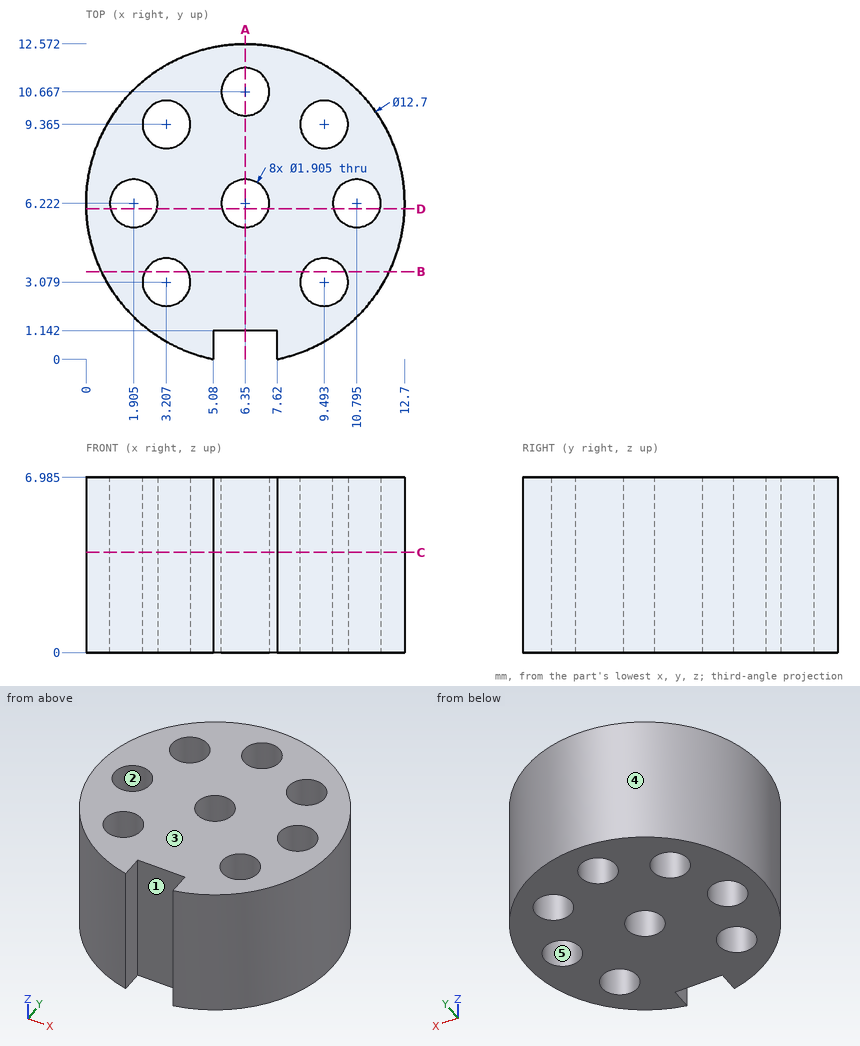
Can you work these out from the drawing? Everything is in mm from the part's minimum corner. A direction names the side the tool comes from. Give positions to 0.01 mm unless a question says otherwise; leave off trailing zeros. Order: outer loops, then holes, each group sorted by start corner. A loop starts at its lowest first (then second) coordinate and runs counter-clockwise, first axis right, second up. Notation, with made-up numbers: M 47.25,32.5 L 80.25,32.5 A19 ccw 80.25,59.5 Z; hole C 28,10 d4. An arc over 180 degrees is marked long. One line per question, with ' | ' between items.
1. For the marked faces 1 and 2, which set-ups out of +Z, -Z, +X, -X, +Y, -Y let a thin tool reach every point of the face, with its end or its side?
Results:
face 1: +Z, -Z, -Y | face 2: +Z, -Z
2. I want a section at C-C (z = 4). Give the number of separate pieces and of enclosed holes in the cut face, and give its area (3 significant figures).
Results:
separate pieces: 1 | enclosed holes: 8 | area: 101 mm²
3. We'd pull the mould along X, two halves only. Please class the marked faces 3, 4 and 5: +X half, -X half, draft (parallel to the pull), parting line (faces both ways), or undercut.
Results:
face 3: draft | face 4: parting line | face 5: undercut
4. If I drill on line 1 (Y direction, x = 6.35, z = 2) (1 decimal); line 2 (X direction, y = 6.25, z = 2); line 3 (X direction, y = 8.5, z = 3.5) (1 decimal), over which ranges is the centre line in solid material (lowest first)?
Results:
line 1: 1.1 to 5.3, 7.2 to 9.7, 11.6 to 12.6 | line 2: 0 to 0.95, 2.86 to 5.4, 7.3 to 9.84, 11.75 to 12.7 | line 3: 0.4 to 2.8, 3.6 to 9.1, 9.9 to 12.3
5. I want a section at A-A (x = 6.35). List the corners of the cut face in (y, z) for me (1 decimal).
Results:
outline: M 1.1,0 L 5.3,0 L 5.3,7 L 1.1,7 Z; M 7.2,0 L 9.7,0 L 9.7,7 L 7.2,7 Z; M 11.6,0 L 12.6,0 L 12.6,7 L 11.6,7 Z
6. I want a section at D-D (y = 6). List the corners of the cut face in (x, z) for me (1 decimal).
Results:
outline: M 0,0 L 1,0 L 1,7 L 0,7 Z; M 2.8,0 L 5.4,0 L 5.4,7 L 2.8,7 Z; M 7.3,0 L 9.9,0 L 9.9,7 L 7.3,7 Z; M 11.7,0 L 12.7,0 L 12.7,7 L 11.7,7 Z
7. I want a section at B-B (y = 3.5). List the corners of the cut face in (x, z) for me (1 decimal).
Results:
outline: M 0.6,0 L 2.4,0 L 2.4,7 L 0.6,7 Z; M 4.1,0 L 8.6,0 L 8.6,7 L 4.1,7 Z; M 10.3,0 L 12.1,0 L 12.1,7 L 10.3,7 Z
8. I'm going to push flat-ended pins straight in: pin 1 (0.9 mm diameter, centred on y = 0.5, z = 2.5, fed in from -X); pin 2 (0.9 mm diameter, centred on y = 0.5, z = 2, fed in from +X); pin 3 (2 mm diameter, centred on x = 6.5, z = 5, fed in from -Y). Where does each tip first touch, or does it pass through?
Results:
pin 1: x = 2.81 | pin 2: x = 9.89 | pin 3: y = 1.14
